Design review of the part built by this model. Coordinates are the model's own, in mm. Face numbers are marked on the shaded views. A direction names the side the tool comes from. Coordinates: 2 decimals unless noted, no trailing zeros. Loops run counter-clockwise (first coordinate to the right, second up) from the corner with the lowest first, then second, coordinate; pieces in that order, holes last.
from build123d import *

# Parameters (mm, degrees)
F0_W     = 132
F0_H     = 66.5
F0_W_2   = 10
F0_H_2   = 21
F0_W_3   = 40
F0_H_3   = 35.5
F1_DEPTH = 17
F2_W     = 132
F2_H     = 66.5
F2_W_2   = 10
F2_H_2   = 21
F2_W_3   = 40
F2_H_3   = 35.5
F3_DEPTH = 3
F5_DEPTH = 3
F6_ANGLE = 180
F7_R     = 4
F8_R     = 2
F9_SIZE  = 1
F10_SIZE = 1


with BuildPart() as f1:
    # F0 (on Top) → F1 (new body)
    with BuildSketch(Plane.XY):
        with Locations((-10.436555624, -5.9587561041)):
            Rectangle(F0_W, F0_H)
        with Locations((-62.436555624, -24.7087561041)):
            Rectangle(F0_W_2, F0_H_2, mode=Mode.SUBTRACT)
        with Locations((-44.436555624, -24.7087561041)):
            Rectangle(F0_W_2, F0_H_2, mode=Mode.SUBTRACT)
        with Locations((-19.436555624, -24.7087561041)):
            Rectangle(F0_W_2, F0_H_2, mode=Mode.SUBTRACT)
        with Locations((-1.436555624, -24.7087561041)):
            Rectangle(F0_W_2, F0_H_2, mode=Mode.SUBTRACT)
        with Locations((23.563444376, -24.7087561041)):
            Rectangle(F0_W_2, F0_H_2, mode=Mode.SUBTRACT)
        with Locations((41.563444376, -24.7087561041)):
            Rectangle(F0_W_2, F0_H_2, mode=Mode.SUBTRACT)
        with Locations((-53.436555624, 6.5412438959)):
            Rectangle(F0_W_3, F0_H_3, mode=Mode.SUBTRACT)
        with Locations((-10.436555624, 6.5412438959)):
            Rectangle(F0_W_3, F0_H_3, mode=Mode.SUBTRACT)
        with Locations((32.563444376, 6.5412438959)):
            Rectangle(F0_W_3, F0_H_3, mode=Mode.SUBTRACT)
    extrude(amount=F1_DEPTH)

    # F2 (on face) → F3 (join)
    with BuildSketch(Plane.XY.offset(17)):
        with Locations((-10.436555624, -5.9587561041)):
            Rectangle(F2_W, F2_H)
        with Locations((-62.436555624, -24.7087561041)):
            Rectangle(F2_W_2, F2_H_2, mode=Mode.SUBTRACT)
        with Locations((-44.436555624, -24.7087561041)):
            Rectangle(F2_W_2, F2_H_2, mode=Mode.SUBTRACT)
        with Locations((-19.436555624, -24.7087561041)):
            Rectangle(F2_W_2, F2_H_2, mode=Mode.SUBTRACT)
        with Locations((-1.436555624, -24.7087561041)):
            Rectangle(F2_W_2, F2_H_2, mode=Mode.SUBTRACT)
        with Locations((23.563444376, -24.7087561041)):
            Rectangle(F2_W_2, F2_H_2, mode=Mode.SUBTRACT)
        with Locations((41.563444376, -24.7087561041)):
            Rectangle(F2_W_2, F2_H_2, mode=Mode.SUBTRACT)
        with Locations((-53.436555624, 6.5412438959)):
            Rectangle(F2_W_3, F2_H_3, mode=Mode.SUBTRACT)
        with Locations((-10.436555624, 6.5412438959)):
            Rectangle(F2_W_3, F2_H_3, mode=Mode.SUBTRACT)
        with Locations((32.563444376, 6.5412438959)):
            Rectangle(F2_W_3, F2_H_3, mode=Mode.SUBTRACT)
        with Locations((-53.436555624, 6.5412438959)):
            Rectangle(F2_W_3, F2_H_3)
        with Locations((-10.436555624, 6.5412438959)):
            Rectangle(F2_W_3, F2_H_3)
        with Locations((32.563444376, 6.5412438959)):
            Rectangle(F2_W_3, F2_H_3)
        with Locations((41.563444376, -24.7087561041)):
            Rectangle(F2_W_2, F2_H_2)
        with Locations((23.563444376, -24.7087561041)):
            Rectangle(F2_W_2, F2_H_2)
        with Locations((-1.436555624, -24.7087561041)):
            Rectangle(F2_W_2, F2_H_2)
        with Locations((-19.436555624, -24.7087561041)):
            Rectangle(F2_W_2, F2_H_2)
        with Locations((-44.436555624, -24.7087561041)):
            Rectangle(F2_W_2, F2_H_2)
        with Locations((-62.436555624, -24.7087561041)):
            Rectangle(F2_W_2, F2_H_2)
    extrude(amount=F3_DEPTH)

    # F4 (on face) → F5 (cut, through all)
    with BuildSketch(Plane(origin=(0, 27.2912438959, 0), x_dir=(-1, 0, 0), z_dir=(0, 1, 0))):
        with BuildLine():
            Line((57.436555624, 0), (57.436555624, 7))
            ThreePointArc((57.436555624, 7), (53.436555624, 11), (49.436555624, 7))
            Line((49.436555624, 7), (49.436555624, 0))
            Line((49.436555624, 0), (57.436555624, 0))
        make_face()
        with BuildLine():
            Line((6.436555624, 0), (14.436555624, 0))
            Line((14.436555624, 0), (14.436555624, 7))
            ThreePointArc((14.436555624, 7), (10.436555624, 11), (6.436555624, 7))
            Line((6.436555624, 7), (6.436555624, 0))
        make_face()
        with BuildLine():
            Line((-36.563444376, 0), (-28.563444376, 0))
            Line((-28.563444376, 0), (-28.563444376, 7))
            ThreePointArc((-28.563444376, 7), (-32.563444376, 11), (-36.563444376, 7))
            Line((-36.563444376, 7), (-36.563444376, 0))
        make_face()
    extrude(amount=-F5_DEPTH, mode=Mode.SUBTRACT)


with BuildPart() as f1_1:
    # F6: moved
    add(f1.part.rotate(Axis((-10.436555624, 27.2912438959, 20), (1, 0, 0)), F6_ANGLE))

    # F7
    f7_edges = [f1_1.edges().sort_by_distance(p)[0] for p in [
        (-76.436556, 27.291244, 30),
        (55.563444, 27.291244, 30),
        (55.563444, 93.791244, 30),
        (-76.436556, 93.791244, 30),
    ]]
    fillet(f7_edges, radius=F7_R)

    # F8
    f8_edges = [f1_1.edges().sort_by_distance(p)[0] for p in [
        (-76.436556, 60.541244, 40),
        (-10.436556, 93.791244, 40),
        (-31.936556, 27.291244, 40),
        (11.063444, 27.291244, 40),
    ]]
    fillet(f8_edges, radius=F8_R)

    # F9
    f9_edges = [f1_1.edges().sort_by_distance(p)[0] for p in [
        (-67.436556, 79.291244, 40),
        (-39.436556, 79.291244, 40),
        (-49.436556, 79.291244, 40),
        (-62.436556, 68.791244, 40),
        (-57.436556, 79.291244, 40),
        (-24.436556, 79.291244, 40),
        (-14.436556, 79.291244, 40),
        (-6.436556, 79.291244, 40),
        (3.563444, 79.291244, 40),
        (18.563444, 79.291244, 40),
        (28.563444, 79.291244, 40),
        (36.563444, 79.291244, 40),
        (46.563444, 79.291244, 40),
        (41.563444, 68.791244, 40),
        (23.563444, 68.791244, 40),
        (-1.436556, 68.791244, 40),
        (-19.436556, 68.791244, 40),
        (-44.436556, 68.791244, 40),
        (-44.436556, 89.791244, 40),
        (-62.436556, 89.791244, 40),
        (-19.436556, 89.791244, 40),
        (-1.436556, 89.791244, 40),
        (23.563444, 89.791244, 40),
        (41.563444, 89.791244, 40),
    ]]
    chamfer(f9_edges, length=F9_SIZE)

    # F10
    f10_edges = [f1_1.edges().sort_by_distance(p)[0] for p in [
        (-10.436556, 27.291244, 20),
    ]]
    chamfer(f10_edges, length=F10_SIZE)


solid = f1_1.part
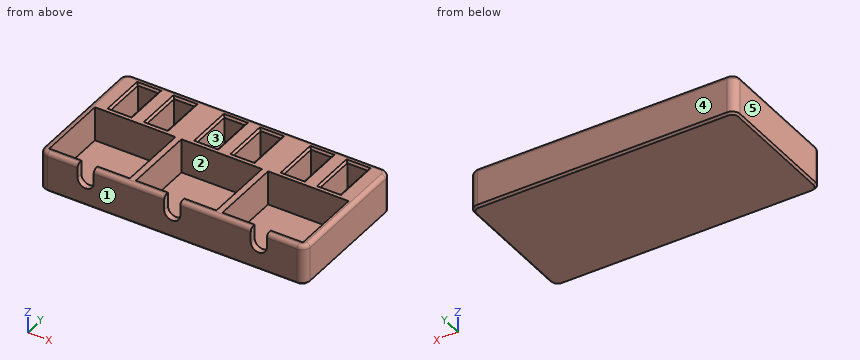
Q1. For line 1 (X direction, y = 52, z = 26.25); line 2 (Y direction, x = 1.5, z = 31.75); line 3 (Y direction, x = -38.5, z = 35.25), list the stretches that pass through material, from the lowest coordinate up.
Q2. Take a section at C-C, the plane z = 25.5. Give the number of separate pieces and of enclosed holes in the cut face, then the cut area to 3 significant figures.
Q3. The part is to be moulded in two halves that separate along Y. For the marked faces 3, 4 and 5, say which applies: pulls with the +Y half, pulls with the -Y half, needs draft (parallel to the pull), parting line crosses it, or undercut.
Q4. Clearance check with flat-ended pins moving along their axes: pin 1 Ø3 at (x, y) = (-17.5, 70.5) entering from +Z; pin 2 Ø3.5 at (y, z) = (29, 37) entering from +X. State where each tip first meets the part, or that it passes through.
Q5. Take a section at D-D, the plane x = -54. Write out the cut boundary in (y, z).
Q6. Take a section at B-B, the plane x = -0.5. Write out the cut boundary in (y, z).
Q7. Take a section at A-A, the plane y = 52. Write out the cut boundary in (x, z).
Q8. Machinability: for the marked faces 1 and 2, which of the approach directions +Z, -Z, +X, -X, +Y, -Y give a long, thin tool a straight path to every point of the face, cutting with its end or side? Answer none if there is none.
Entries:
1. line 1: x = -76.44 to -73.44, -33.44 to -30.44, 9.56 to 12.56, 52.56 to 55.56
1. line 2: y = 27.29 to 30.29, 65.79 to 68.79, 89.79 to 93.79
1. line 3: y = 27.29 to 30.29, 65.79 to 93.79
2. separate pieces: 1
2. enclosed holes: 9
2. area: 3,240 mm2
3. face 3: undercut
3. face 4: pulls with the +Y half
3. face 5: needs draft
4. pin 1: stops at z = 23
4. pin 2: stops at x = 55.53
5. outline: (27.29, 21) - (28.29, 20) - (92.79, 20) - (93.79, 21) - (93.79, 38) arc R2 ccw to (91.79, 40) - (65.79, 40) - (65.79, 23) - (30.29, 23) - (30.29, 29.04) - (27.29, 29.04) - close
6. outline: (27.29, 21) - (28.29, 20) - (92.79, 20) - (93.79, 21) - (93.79, 38) arc R2 ccw to (91.79, 40) - (90.79, 40) - (89.79, 39) - (89.79, 23) - (68.79, 23) - (68.79, 39) - (67.79, 40) - (65.79, 40) - (65.79, 23) - (30.29, 23) - (30.29, 40) - (29.29, 40) arc R2 ccw to (27.29, 38) - close
7. outline: (-76.44, 21) - (-75.44, 20) - (54.56, 20) - (55.56, 21) - (55.56, 38) arc R2 ccw to (53.56, 40) - (52.56, 40) - (52.56, 23) - (12.56, 23) - (12.56, 40) - (9.56, 40) - (9.56, 23) - (-30.44, 23) - (-30.44, 40) - (-33.44, 40) - (-33.44, 23) - (-73.44, 23) - (-73.44, 40) - (-74.44, 40) arc R2 ccw to (-76.44, 38) - close
8. face 1: +Z, -Z, +X, -X, -Y
8. face 2: +Z
